The listing builds one solid part. Answer for the finished solid, in the listing's coordinates (mm). Give positions to 0.01 mm unless a question says otherwise; leave off trailing zeros. Order: outer loops, then holes, each group sorted by start corner. A loop starts at its lowest first (then second) coordinate and runs counter-clockwise, first axis right, second up.
```python
from build123d import *

# Parameters (mm, degrees)
F0_W     = 39
F0_H     = 40
F0_W_2   = 2
F0_H_2   = 32
F0_W_3   = 3
F0_W_4   = 5
F0_W_5   = 4
F0_W_6   = 2.5
F1_DEPTH = 2
F2_R     = 5


with BuildPart() as f1:
    # F0 (on Top) → F1 (new body)
    with BuildSketch(Plane.XY):
        with Locations((19.5, 20)):
            Rectangle(F0_W, F0_H)
        with Locations((5, 20)):
            Rectangle(F0_W_2, F0_H_2, mode=Mode.SUBTRACT)
        with Locations((8.5, 20)):
            Rectangle(F0_W_3, F0_H_2, mode=Mode.SUBTRACT)
        with Locations((15.5, 20)):
            Rectangle(F0_W_4, F0_H_2, mode=Mode.SUBTRACT)
        Polygon((22, 4), (21, 4), (19.5, 4), (19.5, 36), (21, 36), (22, 36), align=None, mode=Mode.SUBTRACT)
        with Locations((26, 20)):
            Rectangle(F0_W_5, F0_H_2, mode=Mode.SUBTRACT)
        with Locations((33.75, 20)):
            Rectangle(F0_W_6, F0_H_2, mode=Mode.SUBTRACT)
    extrude(amount=F1_DEPTH)

    # F2
    f2_edges = [f1.edges().sort_by_distance(p)[0] for p in [
        (39, 40, 1),
        (39, 0, 1),
        (0, 0, 1),
        (0, 40, 1),
    ]]
    fillet(f2_edges, radius=F2_R)


solid = f1.part
```
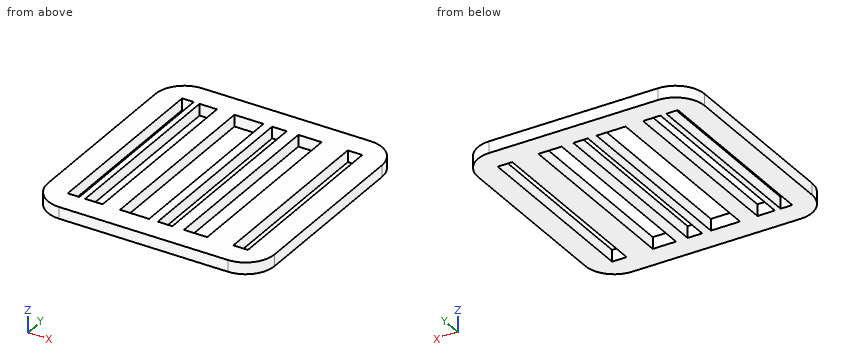
1) Find section B-B (y = 12). Write down the section's boundary in (x, z).
Geometry says:
outline: (0, 0) - (4, 0) - (4, 2) - (0, 2) - close; (6, 0) - (7, 0) - (7, 2) - (6, 2) - close; (10, 0) - (13, 0) - (13, 2) - (10, 2) - close; (18, 0) - (19.5, 0) - (19.5, 2) - (18, 2) - close; (22, 0) - (24, 0) - (24, 2) - (22, 2) - close; (28, 0) - (32.5, 0) - (32.5, 2) - (28, 2) - close; (35, 0) - (39, 0) - (39, 2) - (35, 2) - close
2) Find section A-A (z = 0.85). Count the separate pieces of the cut face and the enclosed holes in it, then the cut area to 3 significant figures.
Geometry says:
separate pieces: 1
enclosed holes: 6
area: 931 mm2
3) Given P1, Ø3, axis at x = 19.5, y = 33.5, coming from the -Z side, flat-ended and moving along its own axis, determine where the tip first touches the part or whether it passes through.
Geometry says:
P1: stops at z = 0
4) Straight lines are drawn through the part: probe 1 along Y at (x, z) = (27.5, 1.5); probe 2 along X at (y, z) = (38, 0.7); probe 3 along Y at (x, z) = (3, 1). For each, find the intervals that lie inside material, in ascending order.
Geometry says:
probe 1: y = 0 to 4, 36 to 40
probe 2: x = 1 to 38
probe 3: y = 0.42 to 39.58
5) Find section C-C (y = 37). Write down the section's boundary in (x, z).
Geometry says:
outline: (0.42, 0) - (38.58, 0) - (38.58, 2) - (0.42, 2) - close
